Design review of the part built by this model. Coordinates are the model's own, in mm. Face numbers are marked on the shaded views. A direction names the side the tool comes from. Round coordinates to 2 decimals unless told otherwise and drop trailing zeros. Order: outer loops, then holes, each group sorted by start corner. A loop starts at its lowest first (then second) coordinate and runs counter-clockwise, first axis right, second up.
from build123d import *

# Parameters (mm, degrees)
EXTRUDE_1_DEPTH     = 7.5
SKETCH_2_OUTSIDE_W  = 85.93
SKETCH_2_OUTSIDE_H  = 81.288
SKETCH_2_OUTSIDE_R  = 15
CUT_EXTRUDE_1_DEPTH = 20
CUT_EXTRUDE_1_DRAFT = -45
SKETCH_3_OUTSIDE_W  = 85.93
SKETCH_3_OUTSIDE_H  = 81.288
SKETCH_3_OUTSIDE_R  = 15
CUT_EXTRUDE_2_DEPTH = 20
CUT_EXTRUDE_2_DRAFT = -45
SKETCH_4_R          = 12.5
EXTRUDE_2_DEPTH     = 25
SKETCH_5_R          = 10
CUT_EXTRUDE_3_DEPTH = 17.5
SKETCH_6_R          = 9.585
EXTRUDE_3_DEPTH     = 14.3775
CHAMFER_1_SIZE      = 1
FILLET_1_R          = 0.5
SKETCH_7_R          = 7.585
CUT_EXTRUDE_4_DEPTH = 21.8775


with BuildPart() as part:
    # Эскиз1 → Бобышка-Вытянуть1 (new body)
    with BuildSketch(Plane(origin=(0, 0, 0), x_dir=(0, 0, -1), z_dir=(1, 0, 0))):
        Polygon((17.320508076, 0), (8.660254038, 15), (-8.660254038, 15), (-17.320508076, 0), (-8.660254038, -15), (8.660254038, -15), align=None)
    extrude(amount=-EXTRUDE_1_DEPTH)


with BuildPart() as cut_extrude_1_tool:
    # Эскиз2 outside → Вырез-Вытянуть1 (with draft: the straight prism first)
    with BuildSketch(Plane(origin=(0, 0, 0), x_dir=(0, 0, -1), z_dir=(1, 0, 0))):
        Rectangle(SKETCH_2_OUTSIDE_W, SKETCH_2_OUTSIDE_H)
        Circle(SKETCH_2_OUTSIDE_R, mode=Mode.SUBTRACT)
    extrude(amount=-CUT_EXTRUDE_1_DEPTH)
    # Вырез-Вытянуть1: the draft: its side faces are tilted about the plane it starts from
    cut_extrude_1_sides = [cut_extrude_1_tool.faces().sort_by_distance(p)[0] for p in [
        (-10, -40.644, 0),
        (-10, 0, -42.965),
        (-10, 40.644, 0),
        (-10, 0, 42.965),
        (-10, 0, 15),
    ]]
    draft(cut_extrude_1_sides, Plane(origin=(0, 0, 0), x_dir=(0, 0, -1), z_dir=(1, 0, 0)), CUT_EXTRUDE_1_DRAFT)


with BuildPart() as part_1:
    add(part.part)

    # Вырез-Вытянуть1: cut by cut_extrude_1_tool
    add(cut_extrude_1_tool.part, mode=Mode.SUBTRACT)


with BuildPart() as cut_extrude_2_tool:
    # Эскиз3 outside → Вырез-Вытянуть2 (with draft: the straight prism first)
    with BuildSketch(Plane.ZY.offset(7.5)):
        Rectangle(SKETCH_3_OUTSIDE_W, SKETCH_3_OUTSIDE_H)
        Circle(SKETCH_3_OUTSIDE_R, mode=Mode.SUBTRACT)
    extrude(amount=-CUT_EXTRUDE_2_DEPTH)
    # Вырез-Вытянуть2: the draft: its side faces are tilted about the plane it starts from
    cut_extrude_2_sides = [cut_extrude_2_tool.faces().sort_by_distance(p)[0] for p in [
        (2.5, -40.644, 0),
        (2.5, 0, 42.965),
        (2.5, 40.644, 0),
        (2.5, 0, -42.965),
        (2.5, 0, -15),
    ]]
    draft(cut_extrude_2_sides, Plane.ZY.offset(7.5), CUT_EXTRUDE_2_DRAFT)


with BuildPart() as part_2:
    add(part_1.part)

    # Вырез-Вытянуть2: cut by cut_extrude_2_tool
    add(cut_extrude_2_tool.part, mode=Mode.SUBTRACT)

    # Эскиз4 → Бобышка-Вытянуть2 (add)
    with BuildSketch(Plane(origin=(0, 0, 0), x_dir=(0, 0, -1), z_dir=(1, 0, 0))):
        Circle(SKETCH_4_R)
    extrude(amount=-EXTRUDE_2_DEPTH)

    # Эскиз5 → Вырез-Вытянуть3 (cut)
    with BuildSketch(Plane.ZY.offset(25)):
        Circle(SKETCH_5_R)
    extrude(amount=-CUT_EXTRUDE_3_DEPTH, mode=Mode.SUBTRACT)

    # Эскиз6 → Бобышка-Вытянуть3 (add)
    with BuildSketch(Plane(origin=(0, 0, 0), x_dir=(0, 0, -1), z_dir=(1, 0, 0))):
        Circle(SKETCH_6_R)
    extrude(amount=EXTRUDE_3_DEPTH)

    # Фаска1
    chamfer_1_edges = [part_2.edges().sort_by_distance(p)[0] for p in [
        (14.3775, 0, 9.585),
    ]]
    chamfer(chamfer_1_edges, length=CHAMFER_1_SIZE)

    # Скругление1
    fillet_1_edges = [part_2.edges().sort_by_distance(p)[0] for p in [
        (-25, 0, 12.5),
        (-25, 0, -10),
    ]]
    fillet(fillet_1_edges, radius=FILLET_1_R)

    # Эскиз7 → Вырез-Вытянуть4 (cut)
    with BuildSketch(Plane(origin=(14.3775, 0, 0), x_dir=(0, 0, -1), z_dir=(1, 0, 0))):
        Circle(SKETCH_7_R)
    extrude(amount=-CUT_EXTRUDE_4_DEPTH, mode=Mode.SUBTRACT)


solid = part_2.part
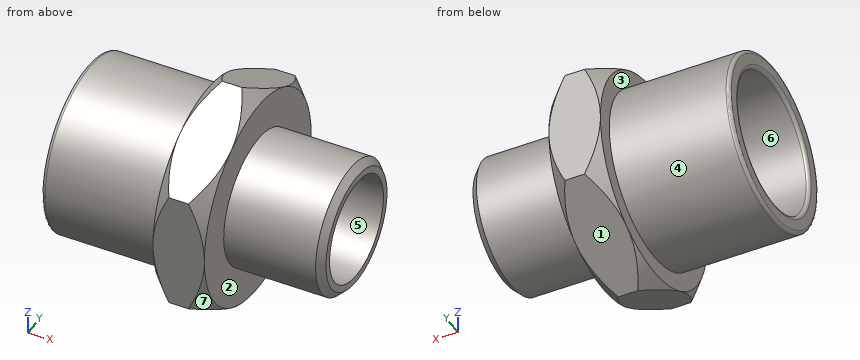
1) To check wall thickness, follow line 1 along Y through (x, z) = (-22, 0); line 2 along Y through (x, z) = (-1.5, 0) (3 decimals); line 3 along X through (y, z) = (-8.5, 10). State the ranges of each line that lie inside material, in increasing order.
Results:
line 1: y = -12.5 to -10, 10 to 12.5
line 2: y = -15 to -7.585, 7.585 to 15
line 3: x = -7.5 to 0
2) Clearance check with flat-ended pins moving along their axes: P1, Ø2, axis at y = -7.5, z = -4.5, coming from the -X side; P2, Ø6, axis at x = -19.5, z = -5.5, coming from the +Y side; P3, Ø12, axis at x = -15.5, z = 6.5, coming from the +Y side. State where each tip first meets the part, or that it passes through.
Results:
P1: stops at x = -7.5
P2: stops at y = 12.25
P3: stops at y = 12.49
3) For the marked faces 1, 2 and 3, list the 3-axis set-ups (+Z, -Z, +X, -X, +Y, -Y) from which the entire face can be reached by the end or side of a thin tool; tool diameter is ignored.
Results:
face 1: -Z, +X, -X, +Y
face 2: +X
face 3: -X
4) Take a section at B-B on x = -9. Give the boundary of the cut face in (y, z).
Results:
outline: circle Ø25 at (0, 0); hole circle Ø20 at (0, 0)
5) The part is to be moulded in two halves that separate along Z. For the marked faces 4, 5, 6 and 7, say which applies: released by +Z, released by -Z, zero draft, split by the parting line, or undercut.
Results:
face 4: split by the parting line
face 5: undercut
face 6: undercut
face 7: released by -Z
6) Take a section at A-A on x = 4.5. Give the boundary of the cut face in (y, z) (3 decimals).
Results:
outline: circle Ø19.17 at (0, 0); hole circle Ø15.17 at (0, 0)
